from build123d import *

# Parameters (mm, degrees)
F0_W     = 160
F0_H     = 300
F1_DEPTH = 10
F3_D     = 5
F3_DEPTH = 10
F3_TIP   = 1.5021515476
F5_D     = 5


with BuildPart() as f1:
    # F0 (on Front) → F1 (new body)
    with BuildSketch(Plane.XZ):
        with Locations((25.1540820301, 94.790057838)):
            Rectangle(F0_W, F0_H)
    extrude(amount=F1_DEPTH)

    # F3
    with Locations(Plane(origin=(0, 0, -55.209942162), x_dir=(1, 0, 0), z_dir=(0, 0, -1))):
        with Locations((-1.1459179699, 5), (51.4540820301, 5)):
            Hole(F3_D / 2, depth=F3_DEPTH)
            with Locations((0, 0, -(F3_DEPTH + F3_TIP / 2))):  # 118° drill point
                Cone(0, F3_D / 2, F3_TIP, mode=Mode.SUBTRACT)

    # F5 (through all)
    with Locations(Plane.XZ.offset(10)):
        with Locations((-43.2748445049, 157.7490222116)):
            Hole(F5_D / 2)


solid = f1.part
Work out the finished part from the listing and answer in its coordinate system (mm). Round coordinates to 2 decimals unless told otherwise and drop trailing zeros. One line per question, with ' | ' between items. Start each with the question number.
(1) For a pull along Z with two mould halves and no side action, classify faces 1 (the face through (24, -5, -55.21)), 2 (the face through (24, -5, 244.79)), 3 (the face through (-54.846, -5, 93)) as released by +Z, released by -Z, zero draft, split by the parting line, or undercut.
(2) Find the intervals of material crossed by line 1 (Z direction, x = -43.5, y = -4.5); line 2 (Z direction, x = -44, y = -1.25), in increasing order.
(3) A flat-ended cylindrical pin translates along its axis: pin 1 Ø4.5 at (x, y) = (-1.15, -5) entering from -Z. Find the tip coordinate at first contact, or state that the pin passes through.
Geometry check:
1) face 1: released by -Z | face 2: released by +Z | face 3: zero draft
2) line 1: z = -55.21 to 155.26, 160.24 to 244.79 | line 2: z = -55.21 to 155.36, 160.14 to 244.79
3) pin 1: stops at z = -45.06
